```python
from build123d import *

# Parameters (mm, degrees)
SKETCH1_W           = 12.7
SKETCH1_H           = 31.75
BOSS_EXTRUDE1_DEPTH = 8.89
SKETCH2_W           = 8.128
SKETCH2_H           = 12.7
CUT_EXTRUDE1_DEPTH  = 8.89


with BuildPart() as part:
    # Sketch1 → Boss-Extrude1 (new body)
    with BuildSketch(Plane(origin=(0, 0, 0), x_dir=(1, 0, 0), z_dir=(0, 1, 0))):
        with Locations((6.35, 15.875)):
            Rectangle(SKETCH1_W, SKETCH1_H)
    extrude(amount=BOSS_EXTRUDE1_DEPTH)

    # Sketch2 → Cut-Extrude1 (cut)
    with BuildSketch(Plane(origin=(0, 8.89, 0), x_dir=(1, 0, 0), z_dir=(0, 1, 0))):
        with Locations((6.35, 25.4)):
            Rectangle(SKETCH2_W, SKETCH2_H)
        with BuildLine():
            ThreePointArc((9.652, 5.08), (8.837060816, 7.252034185), (6.7945, 8.351944949))
            Line((6.7945, 8.351944949), (6.7945, 1.808055051))
            ThreePointArc((6.7945, 1.808055051), (8.837060816, 2.907965815), (9.652, 5.08))
        make_face()
        with BuildLine():
            Line((5.9055, 1.808055051), (5.9055, 8.351944949))
            ThreePointArc((5.9055, 8.351944949), (3.048, 5.08), (5.9055, 1.808055051))
        make_face()
    extrude(amount=-CUT_EXTRUDE1_DEPTH, mode=Mode.SUBTRACT)


solid = part.part
```
The model under review builds one solid part; all positions refer to its coordinate system, in mm. A direction names the side the tool comes from. Round coordinates to 2 decimals unless told otherwise and drop trailing zeros. Loops run counter-clockwise (first coordinate to the right, second up) from the corner with the lowest first, then second, coordinate; pieces in that order, holes last. Notation, with made-up numbers: (-5.5, 7) - (17.5, 7) arc R32 ccw to (17.5, 46) - close; hole circle Ø5 at (72.25, 59.25). An arc over 180 degrees is marked (long way). Use a Markdown table: item, result. Add a question column.
Q1. Add section C-C (x = 4). State the section outline as (y, z) points, plus the area to 3 significant figures.
Q2. Add section D-D (z = -3). State the section outline as (x, y) points.
Q3. Insertion check: pin 1 Ø4 at (x, y) = (8, 6.5) entering from -Z. The pin has a flat end and moves straight along its axis. Give the tip position at first contact, or say it passes through.
Q4. Add section B-B (z = -19.5). State the section outline as (x, y) points.
Q5. Machinability: for faces 4 (the face through (5.906, 5, -5)), 5 (the face through (1, 4, -31.75)), 6 (the face through (6, 5, -19.05)), which of the approach directions +Z, -Z, +X, -X, +Y, -Y give a long, thin tool a straight path to every point of the face, cutting with its end or side? Answer none if there is none.
Q6. Add section A-A (y = 3). State the section outline as (x, z) points, plus the area to 3 significant figures.
Q7. For probe 1 along X at (y, z) = (1.5, -5); probe 2 along X at (y, z) = (1.75, -28.5); probe 3 along X at (y, z) = (4.5, -6), list the stretches that pass through material, from the lowest coordinate up.
Q8. The part is to be moulded in two halves that separate along Z. For faces 1 (the face through (12.7, 4, -16)), 2 (the face through (12, 4, -31.75)), 3 (the face through (3.05, 4.51, -5.15)), say which applies: pulls with the +Z half, pulls with the -Z half, needs draft (parallel to the pull), parting line crosses it, or undercut.
Worked answers:
| question | item | result |
|---|---|---|
| 1 | outline | (0, -19.05) - (8.89, -19.05) - (8.89, -7.4) - (0, -7.4) - close; (0, -2.76) - (8.89, -2.76) - (8.89, 0) - (0, 0) - close |
| 1 | area | 128 mm² |
| 2 | outline | (0, 0) - (3.79, 0) - (3.79, 8.89) - (0, 8.89) - close; (5.91, 0) - (6.79, 0) - (6.79, 8.89) - (5.91, 8.89) - close; (8.91, 0) - (12.7, 0) - (12.7, 8.89) - (8.91, 8.89) - close |
| 3 | pin 1 | z = -19.05 |
| 4 | outline | (0, 0) - (2.29, 0) - (2.29, 8.89) - (0, 8.89) - close; (10.41, 0) - (12.7, 0) - (12.7, 8.89) - (10.41, 8.89) - close |
| 5 | face 4 | +Y, -Y |
| 5 | face 5 | -Z, +X, -X, +Y, -Y |
| 5 | face 6 | -Z, +Y, -Y |
| 6 | outline | (0, -31.75) - (2.29, -31.75) - (2.29, -19.05) - (10.41, -19.05) - (10.41, -31.75) - (12.7, -31.75) - (12.7, 0) - (0, 0) - close; hole (5.91, -8.35) - (5.91, -1.81) arc R3.3 ccw to start; hole (6.79, -8.35) arc R3.3 ccw to (6.79, -1.81) - close |
| 6 | area | 272 mm² |
| 7 | probe 1 | 0 to 3.05, 5.91 to 6.79, 9.65 to 12.7 |
| 7 | probe 2 | 0 to 2.29, 10.41 to 12.7 |
| 7 | probe 3 | 0 to 3.18, 5.91 to 6.79, 9.52 to 12.7 |
| 8 | face 1 | needs draft |
| 8 | face 2 | pulls with the -Z half |
| 8 | face 3 | undercut |
